Geometry check sheet. Reference: the model listing, model coordinates, mm. Face numbers are marked on the shaded views. A direction names the side the tool comes from. Coordinates: 2 decimals unless noted, no trailing zeros. Write each loop counter-clockwise with the first axis right and the second up, starting at its lowest first coordinate (ties: lowest second). Pieces come first, ordered by that corner, then holes. Notation, with made-up numbers: (-5.75, -17) -> (9.25, -17) arc R5 cw to (9.25, -13) -> close; hole circle Ø5 at (41, 70.5). An arc over 180 degrees is marked (long way). Answer in a Markdown table with one row per item. Add a question column.
Q1. Section check C-C, the plane y = 25. Record the boundary of the cut face in (x, z), and give its area (3 significant figures).
Q2. Gauge pin test, flat ends, axial feed: P1, Ø9.5, axis at x = 10.5, z = -4, coming from the -Y side; P2, Ø1.5, axis at x = 12.5, z = -10, coming from the +Y side; P3, Ø4, axis at x = 10.5, z = -4, coming from the +Y side. Record the tip position at first contact, or that the pin passes through.
Q3. Thickness scan on line 1 (Y direction, x = 1, z = -0.5); line 2 (Z direction, x = 10.5, y = 14.3); line 3 (X direction, y = 14.75, z = -4). Record the ranges inside material, lowest first.
Q4. Section check B-B, the plane z = 0. Record the boundary of the cut face in (x, y).
Q5. Tool access check on the marked faces 1, 2, 3, 4 and 5. Record the directions out of +Z, -Z, +X, -X, +Y, -Y that give a thin tool (end or side, any length) a straight path to the whole face; none if there is none.
Q6. Section check A-A, the plane x = -7. Record the boundary of the cut face in (y, z).
Q7. Section check D-D, the plane x = 4.5. Record the boundary of the cut face in (y, z), and give its area (3 significant figures).
Q8. Release check for a two-part mould opening along Y. For the marked faces 6, 7, 8 and 9 record: pulls with the +Y half, pulls with the -Y half, needs draft (parallel to the pull), parting line crosses it, or undercut.
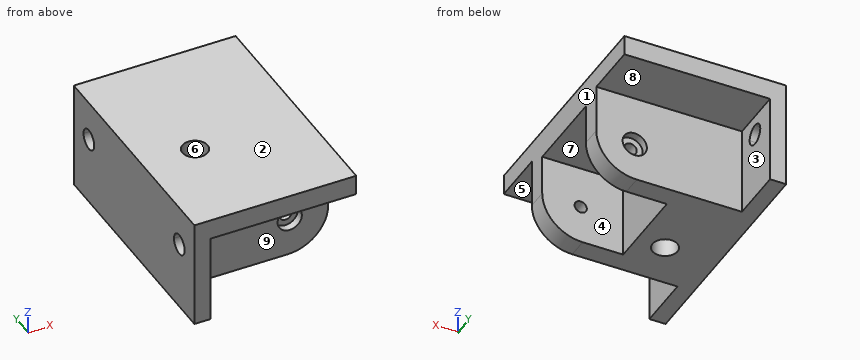
```python
from build123d import *

# Parameters (mm, degrees)
EXTRUDE_1_DEPTH      = 58
SKETCH_2_R           = 3
CUT_EXTRUDE_1_DEPTH  = 58
SKETCH_3_W           = 15
SKETCH_3_H           = 14.5
SKETCH_3_W_2         = 25
CUT_EXTRUDE_2_DEPTH  = 22
SKETCH_5_W           = 4
SKETCH_5_H           = 14.5
EXTRUDE_2_DEPTH      = 22
CUT_EXTRUDE_3_DEPTH  = 22
CUT_EXTRUDE_START    = -30
CUT_EXTRUDE_4_DEPTH  = 30
EXTRUDE_START        = -4
EXTRUDE_5_DEPTH      = 4
EXTRUDE_6_DEPTH      = 4
SKETCH_18_R          = 3.05
CUT_EXTRUDE_7_DEPTH  = 50
SKETCH_17_R          = 1.51
CUT_EXTRUDE_8_DEPTH  = 50
EXTRUDE_7_DEPTH      = 4
EXTRUDE_START_2      = 1
SKETCH_20_R          = 1.51
EXTRUDE_8_DEPTH      = 1
SKETCH_21_R          = 3
SKETCH_21_R_2        = 1.51
CUT_EXTRUDE_9_DEPTH  = 2
EXTRUDE_9_DEPTH      = 4
SKETCH_23_R          = 1.51
EXTRUDE_10_DEPTH     = 1
CUT_EXTRUDE_START_2  = -2
SKETCH_24_R          = 3
CUT_EXTRUDE_10_DEPTH = 2
CUT_EXTRUDE_11_DEPTH = 100
SKETCH_26_R          = 3.05
EXTRUDE_11_DEPTH     = 27
SKETCH_27_R          = 3.1
CUT_EXTRUDE_12_DEPTH = 27
SKETCH_29_W          = 20
SKETCH_29_H          = 21
CUT_EXTRUDE_13_DEPTH = 20
EXTRUDE_START_3      = -5
SKETCH_30_R          = 3
EXTRUDE_12_DEPTH     = 5
SKETCH_32_R          = 3
EXTRUDE_13_DEPTH     = 5
SKETCH_34_R          = 1.51
CUT_EXTRUDE_14_DEPTH = 100
SKETCH_35_R          = 3
CUT_EXTRUDE_15_DEPTH = 2
SKETCH_36_R          = 3
CUT_EXTRUDE_16_DEPTH = 2


with BuildPart() as part:
    # 草图1 → 凸台-拉伸1 (new body)
    with BuildSketch(Plane(origin=(0, 0, 0), x_dir=(1, 0, 0), z_dir=(0, 1, 0))):
        with BuildLine():
            Line((-20, 13.5), (5, 13.5))
            ThreePointArc((5, 13.5), (15.606601718, 9.106601718), (20, -1.5))
            Line((20, -1.5), (20, -13.5))
            Line((20, -13.5), (-20, -13.5))
            Line((-20, -13.5), (-20, 13.5))
        make_face()
    extrude(amount=EXTRUDE_1_DEPTH)

    # 草图2 → 切除-拉伸1 (cut)
    with BuildSketch(Plane.XY.offset(13.5)):
        with Locations((-7, 33)):
            Circle(SKETCH_2_R)
    extrude(amount=-CUT_EXTRUDE_1_DEPTH, mode=Mode.SUBTRACT)

    # 草图3 → 切除-拉伸2 (cut)
    with BuildSketch(Plane(origin=(0, 0, -13.5), x_dir=(-1, 0, 0), z_dir=(0, 0, -1))):
        with Locations((-12.5, 50.75)):
            Rectangle(SKETCH_3_W, SKETCH_3_H)
        with Locations((-12.5, 7.25)):
            Rectangle(SKETCH_3_W, SKETCH_3_H)
        with Locations((7.5, 7.25)):
            Rectangle(SKETCH_3_W_2, SKETCH_3_H)
        with Locations((7.5, 50.75)):
            Rectangle(SKETCH_3_W_2, SKETCH_3_H)
    extrude(amount=-CUT_EXTRUDE_2_DEPTH, mode=Mode.SUBTRACT)

    # 草图5 → 凸台-拉伸2 (add)
    with BuildSketch(Plane(origin=(0, 0, 8.5), x_dir=(-1, 0, 0), z_dir=(0, 0, -1))):
        with Locations((18, 7.25)):
            Rectangle(SKETCH_5_W, SKETCH_5_H)
        with Locations((18, 50.75)):
            Rectangle(SKETCH_5_W, SKETCH_5_H)
    extrude(amount=EXTRUDE_2_DEPTH)

    # 草图8 → 切除-拉伸3 (cut)
    with BuildSketch(Plane.ZY.offset(20)):
        with BuildLine():
            ThreePointArc((6.05, 50.75), (5.303122292, 52.553122292), (3.5, 53.3))
            Line((3.5, 53.3), (3.5, 48.2))
            ThreePointArc((3.5, 48.2), (5.303122292, 48.946877708), (6.05, 50.75))
        make_face()
        with BuildLine():
            Line((3.5, 48.2), (3.5, 53.3))
            ThreePointArc((3.5, 53.3), (0.95, 50.75), (3.5, 48.2))
        make_face()
        with BuildLine():
            ThreePointArc((3.5, 9.8), (0.95, 7.25), (3.5, 4.7))
            Line((3.5, 4.7), (3.5, 9.8))
        make_face()
        with BuildLine():
            Line((3.5, 9.8), (3.5, 4.7))
            ThreePointArc((3.5, 4.7), (5.303122292, 5.446877708), (6.05, 7.25))
            ThreePointArc((6.05, 7.25), (5.303122292, 9.053122292), (3.5, 9.8))
        make_face()
    extrude(amount=-CUT_EXTRUDE_3_DEPTH, mode=Mode.SUBTRACT)

    # 草图10 → 切除-拉伸4 (cut)
    with BuildSketch(Plane(origin=(0, 43.5, 0), x_dir=(1, 0, 0), z_dir=(0, 1, 0)).offset(CUT_EXTRUDE_START)):
        with BuildLine():
            Line((20, -6.5), (20, -1.5))
            ThreePointArc((20, -1.5), (15.606601718, 9.106601718), (5, 13.5))
            Line((5, 13.5), (0, 13.5))
            ThreePointArc((0, 13.5), (5.857864376, -0.642135624), (20, -6.5))
        make_face()
        with BuildLine():
            Line((20, -1.5), (20, 13.5))
            Line((20, 13.5), (5, 13.5))
            ThreePointArc((5, 13.5), (15.606601718, 9.106601718), (20, -1.5))
        make_face()
    extrude(amount=CUT_EXTRUDE_4_DEPTH, mode=Mode.SUBTRACT)

    # 草图11 → 凸台-拉伸5 (add)
    with BuildSketch(Plane(origin=(0, 43.5, 0), x_dir=(1, 0, 0), z_dir=(0, 1, 0)).offset(EXTRUDE_START)):
        with BuildLine():
            Line((5, 13.5), (0, 13.5))
            ThreePointArc((0, 13.5), (5.857864376, -0.642135624), (20, -6.5))
            Line((20, -6.5), (20, -1.5))
            ThreePointArc((20, -1.5), (15.606601718, 9.106601718), (5, 13.5))
        make_face()
    extrude(amount=EXTRUDE_5_DEPTH)

    # 草图13 → 凸台-拉伸6 (add)
    with BuildSketch(Plane.XZ.offset(-14.5)):
        with BuildLine():
            Line((0, -13.5), (5, -13.5))
            ThreePointArc((5, -13.5), (15.606601718, -9.106601718), (20, 1.5))
            Line((20, 1.5), (20, 6.5))
            ThreePointArc((20, 6.5), (5.857864376, 0.642135624), (0, -13.5))
        make_face()
    extrude(amount=-EXTRUDE_6_DEPTH)

    # 草图18 → 切除-拉伸7 (cut)
    with BuildSketch(Plane.XY.offset(13.5)):
        with Locations((-7, 33)):
            Circle(SKETCH_18_R)
    extrude(amount=-CUT_EXTRUDE_7_DEPTH, mode=Mode.SUBTRACT)

    # 草图17 → 切除-拉伸8 (cut)
    with BuildSketch(Plane(origin=(0, 43.5, 0), x_dir=(1, 0, 0), z_dir=(0, 1, 0))):
        with Locations(Location((12.928932188, 6.428932188, 0), (0, 0, 270))):
            Circle(SKETCH_17_R)
    extrude(amount=-CUT_EXTRUDE_8_DEPTH, mode=Mode.SUBTRACT)

    # 草图19 → 凸台-拉伸7 (add)
    with BuildSketch(Plane(origin=(0, 43.5, 0), x_dir=(1, 0, 0), z_dir=(0, 1, 0)).offset(EXTRUDE_START)):
        with BuildLine():
            Line((10, 13.5), (5, 13.5))
            ThreePointArc((5, 13.5), (15.606601718, 9.106601718), (20, -1.5))
            Line((20, -1.5), (20, 3.5))
            ThreePointArc((20, 3.5), (17.071067812, 10.571067812), (10, 13.5))
        make_face()
    extrude(amount=EXTRUDE_7_DEPTH)

    # 草图20 → 凸台-拉伸8 (add)
    with BuildSketch(Plane(origin=(0, 43.5, 0), x_dir=(1, 0, 0), z_dir=(0, 1, 0)).offset(EXTRUDE_START_2)):
        with BuildLine():
            Line((20, 3.5), (20, -8.5))
            Line((20, -8.5), (-16, -8.5))
            Line((-16, -8.5), (-16, 13.5))
            Line((-16, 13.5), (10, 13.5))
            ThreePointArc((10, 13.5), (17.071067812, 10.571067812), (20, 3.5))
        make_face()
        with Locations(Location((12.928932188, 6.428932188, 0), (0, 0, 270))):
            Circle(SKETCH_20_R, mode=Mode.SUBTRACT)
    extrude(amount=-EXTRUDE_8_DEPTH)

    # 草图21 → 切除-拉伸9 (cut)
    with BuildSketch(Plane(origin=(0, 44.5, 0), x_dir=(1, 0, 0), z_dir=(0, 1, 0))):
        with Locations(Location((12.928932188, 6.428932188, 0), (0, 0, 270))):
            Circle(SKETCH_21_R)
        with Locations(Location((12.928932188, 6.428932188, 0), (0, 0, 270))):
            Circle(SKETCH_21_R_2, mode=Mode.SUBTRACT)
    extrude(amount=-CUT_EXTRUDE_9_DEPTH, mode=Mode.SUBTRACT)

    # 草图22 → 凸台-拉伸9 (add)
    with BuildSketch(Plane(origin=(0, 14.5, 0), x_dir=(-1, 0, 0), z_dir=(0, -1, 0))):
        with BuildLine():
            Line((-5, 13.5), (-10, 13.5))
            ThreePointArc((-10, 13.5), (-17.071067812, 10.571067812), (-20, 3.5))
            Line((-20, 3.5), (-20, -1.5))
            ThreePointArc((-20, -1.5), (-15.606601718, 9.106601718), (-5, 13.5))
        make_face()
    extrude(amount=-EXTRUDE_9_DEPTH)

    # 草图23 → 凸台-拉伸10 (add)
    with BuildSketch(Plane(origin=(0, 14.5, 0), x_dir=(-1, 0, 0), z_dir=(0, -1, 0))):
        with BuildLine():
            Line((16, -8.5), (16, 13.5))
            Line((16, 13.5), (-10, 13.5))
            ThreePointArc((-10, 13.5), (-17.071067812, 10.571067812), (-20, 3.5))
            Line((-20, 3.5), (-20, -8.5))
            Line((-20, -8.5), (16, -8.5))
        make_face()
        with Locations(Location((-12.928932188, 6.428932188, 0), (0, 0, 270))):
            Circle(SKETCH_23_R, mode=Mode.SUBTRACT)
    extrude(amount=EXTRUDE_10_DEPTH)

    # 草图24 → 切除-拉伸10 (cut)
    with BuildSketch(Plane(origin=(0, 13.5, 0), x_dir=(-1, 0, 0), z_dir=(0, -1, 0)).offset(CUT_EXTRUDE_START_2)):
        with Locations(Location((-12.928932188, 6.428932188, 0), (0, 0, 270))):
            Circle(SKETCH_24_R)
    extrude(amount=CUT_EXTRUDE_10_DEPTH, mode=Mode.SUBTRACT)

    # 草图25 → 切除-拉伸11 (cut)
    with BuildSketch(Plane.XY.offset(13.5)):
        with BuildLine():
            ThreePointArc((-3.95, 25), (-4.843324317, 27.156675683), (-7, 28.05))
            Line((-7, 28.05), (-7, 21.95))
            ThreePointArc((-7, 21.95), (-4.843324317, 22.843324317), (-3.95, 25))
        make_face()
        with BuildLine():
            Line((-7, 21.95), (-7, 28.05))
            ThreePointArc((-7, 28.05), (-10.05, 25), (-7, 21.95))
        make_face()
    extrude(amount=-CUT_EXTRUDE_11_DEPTH, mode=Mode.SUBTRACT)

    # 草图26 → 凸台-拉伸11 (add)
    with BuildSketch(Plane.XY.offset(13.5)):
        with Locations((-7, 33)):
            Circle(SKETCH_26_R)
    extrude(amount=-EXTRUDE_11_DEPTH)

    # 草图27 → 切除-拉伸12 (cut)
    with BuildSketch(Plane.XY.offset(13.5)):
        with Locations((-7, 25)):
            Circle(SKETCH_27_R)
    extrude(amount=-CUT_EXTRUDE_12_DEPTH, mode=Mode.SUBTRACT)

    # 草图29 → 切除-拉伸13 (cut)
    with BuildSketch(Plane(origin=(0, 0, -13.5), x_dir=(-1, 0, 0), z_dir=(0, 0, -1))):
        with Locations((-10, 29)):
            Rectangle(SKETCH_29_W, SKETCH_29_H)
    extrude(amount=-CUT_EXTRUDE_13_DEPTH, mode=Mode.SUBTRACT)

    # 草图30 → 凸台-拉伸12 (add)
    with BuildSketch(Plane(origin=(0, 13.5, 0), x_dir=(-1, 0, 0), z_dir=(0, -1, 0)).offset(EXTRUDE_START_3)):
        with Locations(Location((-12.928932188, 6.428932188, 0), (0, 0, 270))):
            Circle(SKETCH_30_R)
    extrude(amount=EXTRUDE_12_DEPTH)

    # 草图32 → 凸台-拉伸13 (add)
    with BuildSketch(Plane(origin=(0, 44.5, 0), x_dir=(1, 0, 0), z_dir=(0, 1, 0))):
        with Locations((12.928932188, 6.428932188)):
            Circle(SKETCH_32_R)
    extrude(amount=-EXTRUDE_13_DEPTH)

    # 草图34 → 切除-拉伸14 (cut)
    with BuildSketch(Plane(origin=(0, 44.5, 0), x_dir=(1, 0, 0), z_dir=(0, 1, 0))):
        with Locations(Location((10.5, 4, 0), (0, 0, 270))):
            Circle(SKETCH_34_R)
    extrude(amount=-CUT_EXTRUDE_14_DEPTH, mode=Mode.SUBTRACT)

    # 草图35 → 切除-拉伸15 (cut)
    with BuildSketch(Plane(origin=(0, 44.5, 0), x_dir=(1, 0, 0), z_dir=(0, 1, 0))):
        with Locations(Location((10.5, 4, 0), (0, 0, 270))):
            Circle(SKETCH_35_R)
    extrude(amount=-CUT_EXTRUDE_15_DEPTH, mode=Mode.SUBTRACT)

    # 草图36 → 切除-拉伸16 (cut)
    with BuildSketch(Plane(origin=(0, 13.5, 0), x_dir=(-1, 0, 0), z_dir=(0, -1, 0)).offset(CUT_EXTRUDE_START_2)):
        with Locations(Location((-10.5, 4, 0), (0, 0, 270))):
            Circle(SKETCH_36_R)
    extrude(amount=CUT_EXTRUDE_16_DEPTH, mode=Mode.SUBTRACT)


solid = part.part
```
Calculated:
| question | item | result |
|---|---|---|
| 1 | outline | (-20, -13.5) -> (-10.1, -13.5) -> (-10.1, 13.5) -> (-20, 13.5) -> close; (-3.9, -13.5) -> (0, -13.5) -> (0, 6.5) -> (20, 6.5) -> (20, 13.5) -> (-3.9, 13.5) -> close |
| 1 | area | 513 mm² |
| 2 | P1 | stops at y = 13.5 |
| 2 | P2 | stops at y = 44.5 |
| 2 | P3 | stops at y = 42.5 |
| 3 | line 1 | y = 13.5 to 18.5, 39.5 to 44.5 |
| 3 | line 2 | z = -13.49 to -7, -1 to 13.5 |
| 3 | line 3 | x = -20 to 7.5, 13.5 to 19.99 |
| 4 | outline | (-20, 0) -> (-16, 0) -> (-16, 13.5) -> (20, 13.5) -> (20, 18.5) -> (0, 18.5) -> (0, 39.5) -> (20, 39.5) -> (20, 44.5) -> (-16, 44.5) -> (-16, 58) -> (-20, 58) -> close; hole circle Ø6.2 at (-7, 25) |
| 5 | face 1 | +Z, -Z, +X, +Y, -Y |
| 5 | face 2 | +Z, +X, -X, +Y, -Y |
| 5 | face 3 | -Z, +X, +Y |
| 5 | face 4 | -Z, +X |
| 5 | face 5 | -Z, +X, -Y |
| 6 | outline | (0, 8.5) -> (13.5, 8.5) -> (13.5, -13.5) -> (21.9, -13.5) -> (21.9, 13.5) -> (0, 13.5) -> close; (28.1, -13.5) -> (44.5, -13.5) -> (44.5, 8.5) -> (58, 8.5) -> (58, 13.5) -> (28.1, 13.5) -> close |
| 7 | outline | (0, 8.5) -> (13.5, 8.5) -> (13.5, -13.5) -> (18.5, -13.5) -> (18.5, 6.5) -> (39.5, 6.5) -> (39.5, -13.5) -> (44.5, -13.5) -> (44.5, 8.5) -> (58, 8.5) -> (58, 13.5) -> (0, 13.5) -> close |
| 7 | area | 552 mm² |
| 8 | face 6 | undercut |
| 8 | face 7 | undercut |
| 8 | face 8 | needs draft |
| 8 | face 9 | pulls with the -Y half |
